Autodesk Inventor part; units mm, degrees
ref_plane "YZ Plane" through (0, 0, 0) normal (1, 0, 0) x (0, 1, 0)
ref_plane "XZ Plane" through (0, 0, 0) normal (0, 1, 0) x (-1, 0, 0)
ref_plane "XY Plane" through (0, 0, 0) normal (0, 0, 1) x (1, 0, 0)
sketch "Sketch1" plane through (0, 0, 0) normal (0, 0, 1) x (1, 0, 0)
  line L0 (0, 0) -> (0, -45)
  line L1 (0, -45) -> (30, -45)
  line L2 (30, -45) -> (30, 0)
  line L3 (30, 0) -> (0, 0)
  dimension "d0" = 45
  dimension "d1" = 30
extrude "Extrusion1" add sketch "Sketch1" against normal blind 10
sketch "Sketch2" plane through (0, 0, -10) normal (0, 0, -1) x (-1, 0, 0)
  line L0 (0, 0) -> (-30, 0)
  line L1 (-15, 0) -> (-15, -45)
  line L2 (-30, -45) -> (0, -45)
  line L3 (0, -45) -> (0, 0)
  line L4 (0, -22.5) -> (-30, -22.5)
  line L5 (-30, 0) -> (-30, -45)
  circle A0 centre (-15, -15) radius 5
  dimension "d4" = 10
  dimension "d5" = 15
extrude "Extrusion2" add sketch "Sketch2" along normal blind 5 contours A0 L1 | L1 A0
ref_plane "Work Plane1" through (0, -15, 0) normal (0, 1, 0) x (1, 0, 0)
properties part number "esp32CAM"
Can you work these out from the model? Positions are in its coordinate system, mm. A direction names the side the tool comes from. Coordinates: 2 decimals unless noted, no trailing zeros. Write each loop counter-clockwise with the first axis right and the second up, starting at its lowest first coordinate (ties: lowest second). Pieces come first, ordered by that corner, then holes. Notation, with made-up numbers: (6.25, -0.75) - (45.25, -0.75) arc R26 cw to (45.25, 32.25) - close; hole circle Ø1 at (72, -27.5). An arc over 180 degrees is marked (long way). Return JSON: item names as keys, results as strings. Group by question number.
Item 1: I'm going to push a flat-ended pin straight in: pin 1 Ø6 at (x, y) = (3.5, -28.5) entering from -Z. Where does the tip first touch, or does it pass through?
Item 2: If we section it at A-A (y = -15): Write out the boundary of the cut face in (x, z), then the cut area to 3 significant figures.
Item 3: Please list where these lines run through material, in increasing order: probe 1 along Z at (x, y) = (4.5, -35); probe 2 along X at (y, z) = (-14, -12.5); probe 3 along X at (y, z) = (-10.5, -10.75).
Item 4: If we section it at D-D (x = 6.75): Write out the boundary of the cut face in (y, z), then the cut area to 3 significant figures.
Item 5: If we section it at C-C (z = -10.5): Write out the boundary of the cut face in (x, y).
Item 6: If we section it at B-B (x = 15): Write out the boundary of the cut face in (y, z).
Item 7: Which directions (+Z, -Z, +X, -X, +Y, -Y) give clear straight access to the entire face, cutting with the end or side of a thin tool? Please do faces 1 (the face through (16.08, -10.12, -12.46)), 2 (the face through (0, -22, -5)).
Return value:
{
 "1": {"pin 1": "stops at z = -10"},
 "2": {"outline": "(0, -10) - (10, -10) - (10, -15) - (20, -15) - (20, -10) - (30, -10) - (30, 0) - (0, 0) - close", "area": "350 mm^2"},
 "3": {"probe 1": "z = -10 to 0", "probe 2": "x = 10.1 to 19.9", "probe 3": "x = 12.82 to 17.18"},
 "4": {"outline": "(-45, -10) - (0, -10) - (0, 0) - (-45, 0) - close", "area": "450 mm^2"},
 "5": {"outline": "circle Ø10 at (15, -15)"},
 "6": {"outline": "(-45, -10) - (-20, -10) - (-20, -15) - (-10, -15) - (-10, -10) - (0, -10) - (0, 0) - (-45, 0) - close"},
 "7": {"face 1": "-Z", "face 2": "+Z, -Z, -X, +Y, -Y"}
}
